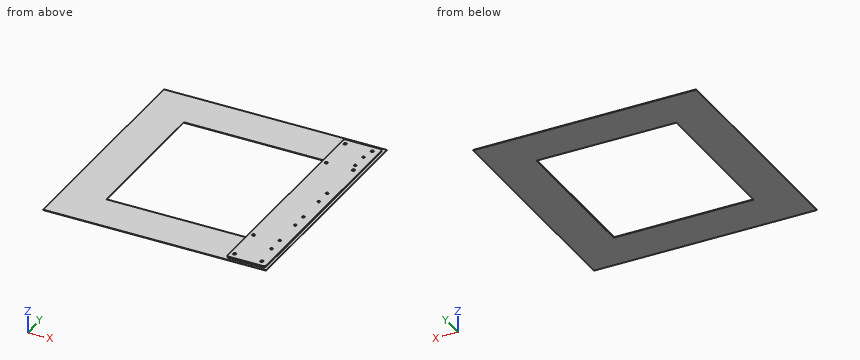
```python
from build123d import *

# Parameters (mm, degrees)
F0_W     = 493
F0_H     = 511
F0_W_2   = 309
F0_H_2   = 327
F1_DEPTH = 1
F2_R     = 3.3
F2_R_2   = 2.75
F3_DEPTH = 3


with BuildPart() as f1:
    # F0 (on Top) → F1 (new body)
    with BuildSketch(Plane.XY):
        with Locations((154.5, 163.5)):
            Rectangle(F0_W, F0_H)
        with Locations((154.5, 163.5)):
            Rectangle(F0_W_2, F0_H_2, mode=Mode.SUBTRACT)
    extrude(amount=F1_DEPTH)

    # F2 (on face) → F3 (join)
    with BuildSketch(Plane.XY.offset(1)):
        with BuildLine():
            Line((390, 412), (315, 412))
            ThreePointArc((315, 412), (311.464466, 410.535534), (310, 407))
            Line((310, 407), (310, -80))
            ThreePointArc((310, -80), (311.464466, -83.535534), (315, -85))
            Line((315, -85), (390, -85))
            ThreePointArc((390, -85), (393.535534, -83.535534), (395, -80))
            Line((395, -80), (395, 407))
            ThreePointArc((395, 407), (393.535534, 410.535534), (390, 412))
        make_face()
        with Locations((320, -70)):
            Circle(F2_R, mode=Mode.SUBTRACT)
        with Locations((380, -70)):
            Circle(F2_R, mode=Mode.SUBTRACT)
        with Locations((320, 10)):
            Circle(F2_R, mode=Mode.SUBTRACT)
        with Locations((375, -19.5)):
            Circle(F2_R_2, mode=Mode.SUBTRACT)
        with Locations((375, 15.5)):
            Circle(F2_R_2, mode=Mode.SUBTRACT)
        with Locations((375, 80.5)):
            Circle(F2_R_2, mode=Mode.SUBTRACT)
        with Locations((375, 115.5)):
            Circle(F2_R_2, mode=Mode.SUBTRACT)
        with Locations((375, 180.5)):
            Circle(F2_R_2, mode=Mode.SUBTRACT)
        with Locations((375, 215.5)):
            Circle(F2_R_2, mode=Mode.SUBTRACT)
        with Locations((320, 317)):
            Circle(F2_R, mode=Mode.SUBTRACT)
        with Locations((380, 317)):
            Circle(F2_R, mode=Mode.SUBTRACT)
        with Locations((375, 334.5)):
            Circle(F2_R_2, mode=Mode.SUBTRACT)
        with Locations((320, 397)):
            Circle(F2_R, mode=Mode.SUBTRACT)
        with Locations((375, 369.5)):
            Circle(F2_R_2, mode=Mode.SUBTRACT)
        with Locations((380, 397)):
            Circle(F2_R, mode=Mode.SUBTRACT)
    extrude(amount=F3_DEPTH)


solid = f1.part
```
Input: part model. Units: mm. Frame: model coordinates. Give positions to 0.01 mm unless a question says otherwise; leave off trailing zeros. Order: outer loops, then holes, each group sorted by start corner. A loop starts at its lowest first (then second) coordinate and runs counter-clockwise, first axis right, second up. Notation, with made-up numbers: M -7,22.5 L 28,22.5 A20 ccw 28,46.5 Z; hole C 48,-8 d1. An arc over 180 degrees is marked long. Return JSON: item names as keys, results as strings.
Item 1: Cut plane D-D (x = -56.5). Return loops of the section in (y, z).
Solutions:
{"outline": "M -92,0 L 419,0 L 419,1 L -92,1 Z"}
Item 2: Cut plane B-B (y = 25.5). Return loops of the section in (x, z).
Solutions:
{"outline": "M -92,0 L 0,0 L 0,1 L -92,1 Z; M 309,0 L 401,0 L 401,1 L 395,1 L 395,4 L 310,4 L 310,1 L 309,1 Z"}
Item 3: First-contact query: P1, Ø5, axis at x = 375, y = 115.5, coming from the +Z side; P2, Ø2, axis at y = 349, z = 2.5, coming from the +X side. Flat tips, straight axial feed; report the tip coordinate or a pass-through.
Solutions:
{"P1": "z = 1", "P2": "x = 395"}
Item 4: Cut plane A-A (x = 61.5). Return loops of the section in (y, z).
Solutions:
{"outline": "M -92,0 L 0,0 L 0,1 L -92,1 Z; M 327,0 L 419,0 L 419,1 L 327,1 Z"}
Item 5: Ray query, probe 1 along Y at (x, z) = (320, 2.85); probe 2 along X at (y, z) = (397, 3.15); probe 3 along X at (y, z) = (180.5, 1.7). Return the intervals inside material, ascending.
Solutions:
{"probe 1": "-85 to -73.3, -66.7 to 6.7, 13.3 to 313.7, 320.3 to 393.7, 400.3 to 412", "probe 2": "310 to 316.7, 323.3 to 376.7, 383.3 to 395", "probe 3": "310 to 372.25, 377.75 to 395"}
Item 6: Cut plane C-C (z = 2.35). State how many separate pieces and enclosed holes the cut face has, then the cut area to 3 significant figures.
Solutions:
{"separate pieces": "1", "enclosed holes": "15", "area": "41,800 mm^2"}
